```python
from build123d import *

# Parameters (mm, degrees)
F1_DEPTH = 5.08
F2_R     = 15.24
F3_DEPTH = 25.4
F2_R_2   = 2.54
F4_DEPTH = 25.4


with BuildPart() as f1:
    # F0 (on Top) → F1 (new body)
    with BuildSketch(Plane.XY):
        with BuildLine():
            ThreePointArc((18.445083, 33.3375), (0, 25.4), (-18.445083, 33.3375))
            ThreePointArc((-18.445083, 33.3375), (-32.995568, 19.05), (-38.093663, -0.694839))
            ThreePointArc((-38.093663, -0.694839), (-21.997045, -12.7), (-19.64858, -32.642661))
            ThreePointArc((-19.64858, -32.642661), (0, -38.1), (19.64858, -32.642661))
            ThreePointArc((19.64858, -32.642661), (21.997045, -12.7), (38.093663, -0.694839))
            ThreePointArc((38.093663, -0.694839), (32.995568, 19.05), (18.445083, 33.3375))
        make_face()
    extrude(amount=F1_DEPTH)

    # F2 (on face) → F3 (cut)
    with BuildSketch(Plane.XY.offset(5.08)):
        Circle(F2_R)
    extrude(amount=-F3_DEPTH, mode=Mode.SUBTRACT)

    # F2 (on face) → F4 (cut)
    with BuildSketch(Plane.XY.offset(5.08)):
        with Locations((7.62, -25.4)):
            Circle(F2_R_2)
        with Locations((-7.62, -25.4)):
            Circle(F2_R_2)
        with Locations((-25.807045, 6.100886)):
            Circle(F2_R_2)
        with Locations((-18.187045, 19.299114)):
            Circle(F2_R_2)
        with Locations((18.187045, 19.299114)):
            Circle(F2_R_2)
        with Locations((25.807045, 6.100886)):
            Circle(F2_R_2)
    extrude(amount=-F4_DEPTH, mode=Mode.SUBTRACT)


solid = f1.part
```
Source: CAD feature listing. Evaluate the final solid. Frame: model axes, mm. Coordinates: 2 decimals unless noted, no trailing zeros. Write each loop counter-clockwise with the first axis right and the second up, starting at its lowest first coordinate (ties: lowest second). Pieces come first, ordered by that corner, then holes. Notation, with made-up numbers: M 44.5,88 L 98.5,88 A13 cw 98.5,108 Z; hole C 77,17 d5. An arc over 180 degrees is marked long. Answer as a JSON object with one key per item and string values.
1. Cut plane A-A on x = 0. Output: boundary loops of the cut face in (y, z).
Evaluation:
{"outline": "M -38.1,0 L -15.24,0 L -15.24,5.08 L -38.1,5.08 Z; M 15.24,0 L 25.4,0 L 25.4,5.08 L 15.24,5.08 Z"}
2. Cut plane C-C on y = -3. Output: boundary loops of the cut face in (x, z), plus the area to 3 significant figures.
Evaluation:
{"outline": "M -32.02,0 L -14.94,0 L -14.94,5.08 L -32.02,5.08 Z; M 14.94,0 L 32.02,0 L 32.02,5.08 L 14.94,5.08 Z", "area": "174 mm^2"}
3. Ray query, L1, parallel to X at y = -0.5, z = 1.6; L2, parallel to Y at x = -7.62, z = 3.55; L3, parallel to X at y = 5, z = 0.7. Return the intervals inside material, ascending.
Evaluation:
{"L1": "-38.1 to -15.23, 15.23 to 38.1", "L2": "-37.33 to -27.94, -22.86 to -13.2, 13.2 to 26.57", "L3": "-37.77 to -28.1, -23.52 to -14.4, 14.4 to 23.52, 28.1 to 37.77"}
4. Cut plane B-B on y = -25.4. Output: boundary loops of the cut face in (x, z).
Evaluation:
{"outline": "M -18.59,0 L -10.16,0 L -10.16,5.08 L -18.59,5.08 Z; M -5.08,0 L 5.08,0 L 5.08,5.08 L -5.08,5.08 Z; M 10.16,0 L 18.59,0 L 18.59,5.08 L 10.16,5.08 Z"}
5. Draft query along Y for faces 1 (the cylindrical face through (-20.2, 17.75, 2.58)), 2 (the cylindrical face through (-23.46, 5.13, 2.58)), 3 (the cylindrical face through (-0.3, -38.1, 2.5)), 4 (the cylindrical face through (0.3, 25.4, 2.5)). Return one class per face: released by +Y, released by -Y, zero draft, split by the parting line, or undercut.
Evaluation:
{"face 1": "undercut", "face 2": "undercut", "face 3": "released by -Y", "face 4": "released by +Y"}
6. Cut plane D-D on z = 3.5. Output: boundary loops of the cut face in (x, y), plus the area to 3 significant figures.
Evaluation:
{"outline": "M -38.09,-0.69 A25.4 cw -19.65,-32.64 A38.1 ccw 19.65,-32.64 A25.4 cw 38.09,-0.69 A38.1 ccw 18.45,33.34 A25.4 cw -18.45,33.34 A38.1 ccw Z; hole C -25.81,6.1 d5.08; hole C -18.19,19.3 d5.08; hole C 0,0 d30.48; hole C -7.62,-25.4 d5.08; hole C 7.62,-25.4 d5.08; hole C 18.19,19.3 d5.08; hole C 25.81,6.1 d5.08", "area": "2,750 mm^2"}
7. Contact query for flat-ended pins moving along their axis: P1, Ø4.5, axis at x = -7.62, y = -25.4, coming from the -Z side; P2, Ø1, axis at y = 3, z = 4, coming from the +X side; P3, Ø1, axis at y = 13, z = 2, coming from the +X side. Output: stop coordinate, or through.
Evaluation:
{"P1": "through", "P2": "x = 38.02", "P3": "x = 35.99"}
